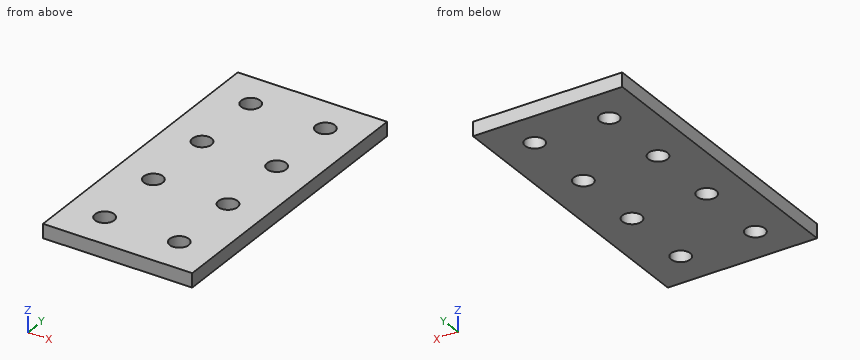
Autodesk Inventor part; units mm, degrees
ref_plane "YZ Plane" through (0, 0, 0) normal (1, 0, 0) x (0, 1, 0)
ref_plane "XZ Plane" through (0, 0, 0) normal (0, 1, 0) x (-1, 0, 0)
ref_plane "XY Plane" through (0, 0, 0) normal (0, 0, 1) x (1, 0, 0)
sketch "Sketch_1" plane through (0, 0, 0) normal (0, 0, 1) x (1, 0, 0)
  line L0 (-25.4, 101.6) -> (-25.4, 0)
  line L1 (-25.4, 0) -> (25.4, 0)
  line L2 (25.4, 0) -> (25.4, 101.6)
  line L3 (25.4, 101.6) -> (-25.4, 101.6)
  circle A0 centre (12.7, 12.7) radius 3.2639
  circle A1 centre (12.7, 38.1) radius 3.2639
  circle A2 centre (12.7, 63.5) radius 3.2639
  circle A3 centre (12.7, 88.9) radius 3.2639
  circle A4 centre (-12.7, 12.7) radius 3.2639
  circle A5 centre (-12.7, 38.1) radius 3.2639
  circle A6 centre (-12.7, 63.5) radius 3.2639
  circle A7 centre (-12.7, 88.9) radius 3.2639
extrude "Extrusion1" add sketch "Sketch_1" along normal blind 4.7752
properties part number "4165"
Model file for the job. Use its own axes, mm. Give positions to 0.01 mm unless a question says otherwise; leave off trailing zeros. Loops run counter-clockwise (first coordinate to the right, second up) from the corner with the lowest first, then second, coordinate; pieces in that order, holes last. Notation, with made-up numbers: (7.25, 89.5) -> (44.25, 89.5) arc R28 cw to (44.25, 123.5) -> close; hole circle Ø7 at (59.25, 74). An arc over 180 degrees is marked (long way). Use a Markdown table: item, result. Add a question column.
(1) Slice it at B-B on x = -12.7. List the corners of the cut face in (y, z), and give its area (3 significant figures).
(2) Drop a flat-ended pin along its axis: pin 1 Ø5 at (x, y) = (-18, 53) entering from -Z. Give the stop position or say it passes through.
(3) Slice it at C-C on z = 1.05. Give the number of separate pieces and of enclosed holes in the cut face, and give its area (3 significant figures).
(4) Slice it at A-A on y = 63.5. List the corners of the cut face in (x, z), and give its area (3 significant figures).
(5) Wall check: line 1 along Y through (x, z) = (12.7, 3.6); line 2 along X through (y, z) = (63, 2.35); line 3 along X through (y, z) = (91.5, 3.9). Give the ranges that are in metal, low to high.
Filled sheet:
| question | item | result |
|---|---|---|
| 1 | outline | (0, 0) -> (9.44, 0) -> (9.44, 4.78) -> (0, 4.78) -> close; (15.96, 0) -> (34.84, 0) -> (34.84, 4.78) -> (15.96, 4.78) -> close; (41.36, 0) -> (60.24, 0) -> (60.24, 4.78) -> (41.36, 4.78) -> close; (66.76, 0) -> (85.64, 0) -> (85.64, 4.78) -> (66.76, 4.78) -> close; (92.16, 0) -> (101.6, 0) -> (101.6, 4.78) -> (92.16, 4.78) -> close |
| 1 | area | 360 mm2 |
| 2 | pin 1 | z = 0 |
| 3 | separate pieces | 1 |
| 3 | enclosed holes | 8 |
| 3 | area | 4,890 mm2 |
| 4 | outline | (-25.4, 0) -> (-15.96, 0) -> (-15.96, 4.78) -> (-25.4, 4.78) -> close; (-9.44, 0) -> (9.44, 0) -> (9.44, 4.78) -> (-9.44, 4.78) -> close; (15.96, 0) -> (25.4, 0) -> (25.4, 4.78) -> (15.96, 4.78) -> close |
| 4 | area | 180 mm2 |
| 5 | line 1 | 0 to 9.44, 15.96 to 34.84, 41.36 to 60.24, 66.76 to 85.64, 92.16 to 101.6 |
| 5 | line 2 | -25.4 to -15.93, -9.47 to 9.47, 15.93 to 25.4 |
| 5 | line 3 | -25.4 to -14.67, -10.73 to 10.73, 14.67 to 25.4 |
